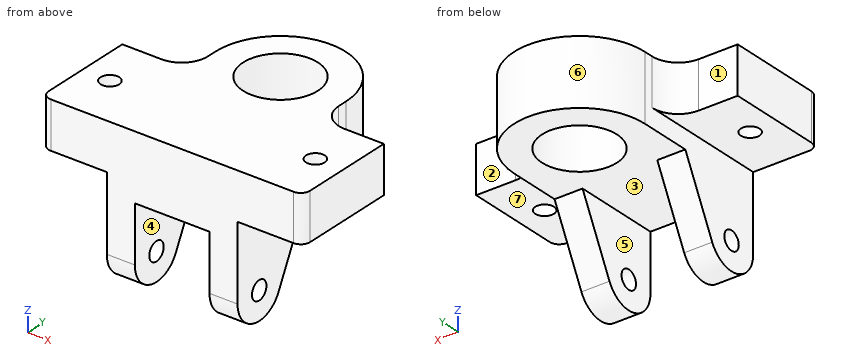
from build123d import *

# Parameters (mm, degrees)
SKETCH1_R           = 5
SKETCH1_R_2         = 20
BOSS_EXTRUDE1_DEPTH = 25
FILLET1_R           = 14
FILLET2_R           = 5
BOSS_EXTRUDE2_START = -10
SKETCH1_3_R         = 20
BOSS_EXTRUDE2_DEPTH = 10
SKETCH3_R           = 5
BOSS_EXTRUDE3_DEPTH = 15


with BuildPart() as part:
    # Sketch1 → Boss-Extrude1 (new body)
    with BuildSketch(Plane.XY):
        with BuildLine():
            Line((-70, 56), (-70, 0))
            Line((-70, 0), (70, 0))
            Line((70, 0), (70, 56))
            Line((70, 56), (35, 56))
            Line((35, 56), (35, 75))
            ThreePointArc((35, 75), (0, 110), (-35, 75))
            Line((-35, 75), (-35, 56))
            Line((-35, 56), (-70, 56))
        make_face()
        with Locations((-55, 28)):
            Circle(SKETCH1_R, mode=Mode.SUBTRACT)
        with Locations((0, 75)):
            Circle(SKETCH1_R_2, mode=Mode.SUBTRACT)
        with Locations((55, 28)):
            Circle(SKETCH1_R, mode=Mode.SUBTRACT)
    extrude(amount=BOSS_EXTRUDE1_DEPTH)

    # Fillet1
    fillet1_edges = [part.edges().sort_by_distance(p)[0] for p in [
        (-35, 56, 12.5),
        (35, 56, 12.5),
    ]]
    fillet(fillet1_edges, radius=FILLET1_R)

    # Fillet2
    fillet2_edges = [part.edges().sort_by_distance(p)[0] for p in [
        (-70, 0, 12.5),
        (70, 0, 12.5),
    ]]
    fillet(fillet2_edges, radius=FILLET2_R)

    # Sketch1_3 → Boss-Extrude2 (add)
    with BuildSketch(Plane.XY.offset(BOSS_EXTRUDE2_START)):
        with BuildLine():
            Line((-35, 56), (-35, 0))
            Line((-35, 0), (35, 0))
            Line((35, 0), (35, 56))
            Line((35, 56), (35, 75))
            ThreePointArc((35, 75), (0, 110), (-35, 75))
            Line((-35, 75), (-35, 56))
        make_face()
        with Locations((0, 75)):
            Circle(SKETCH1_3_R, mode=Mode.SUBTRACT)
    extrude(amount=BOSS_EXTRUDE2_DEPTH)

    # Sketch3 → Boss-Extrude3 (add)
    with BuildSketch(Plane(origin=(35, 0, 0), x_dir=(0, 0, -1), z_dir=(1, 0, 0))):
        with BuildLine():
            Line((10, 47), (10, 0))
            Line((10, 0), (40, 0))
            ThreePointArc((40, 0), (54.590100754, 11.517334354), (46.774992355, 28.382805333))
            Line((46.774992355, 28.382805333), (10, 47))
        make_face()
        with Locations((40, 15)):
            Circle(SKETCH3_R, mode=Mode.SUBTRACT)
    extrude(amount=-BOSS_EXTRUDE3_DEPTH)

    # Mirror1: part across plane


with BuildPart() as part_1:
    add(part.part)
    add(part.part.mirror(Plane(origin=(0, 0, 0), x_dir=(0, 0, 1), z_dir=(1, 0, 0))))


solid = part_1.part
Part model, mm, in its own coordinate system. Face numbers are marked on the shaded views. A direction names the side the tool comes from. Coordinates: 2 decimals unless noted, no trailing zeros. Order: outer loops, then holes, each group sorted by start corner. A loop starts at its lowest first (then second) coordinate and runs counter-clockwise, first axis right, second up.
(1) Tool access for the marked faces 1, 2, 3 and 4: list every direction of +Z, -Z, +X, -X, +Y, -Y with a clear straight run to the whole face (end or side of a thin tool).
Check sheet entries:
face 1: +Z, -Z, -X, +Y
face 2: +Z, -Z, +X, +Y
face 3: -Z, +Y
face 4: -Z, +Y, -Y
(2) Pull direction X, two halves, no side cores. Call the marked faces 5, 6 and 7: pulls with the +X half, pulls with the -X half, needs draft (parallel to the pull), parting line crosses it, or undercut.
Check sheet entries:
face 5: undercut
face 6: parting line crosses it
face 7: needs draft
(3) Slice it at D-D, the plane z = -3. Write the cut outline in (x, y), and give its area (3 significant figures).
Check sheet entries:
outline: (-35, 0) - (35, 0) - (35, 75) arc R35 ccw to (-35, 75) - close; hole circle Ø40 at (0, 75)
area: 5,920 mm2
(4) Slice it at B-B, the plane y = 15. Write the cut outline in (x, z).
Check sheet entries:
outline: (-70, 0) - (-35, 0) - (-35, -35) - (-20, -35) - (-20, -10) - (20, -10) - (20, -35) - (35, -35) - (35, 0) - (70, 0) - (70, 25) - (-70, 25) - close; (-35, -55) - (-20, -55) - (-20, -45) - (-35, -45) - close; (20, -55) - (35, -55) - (35, -45) - (20, -45) - close
(5) Pin check, flat tips, straight feed: pin 1 Ø10.5 at (x, z) = (64, 18.5) entering from +Y; pin 2 Ø10.5 at (x, y) = (58, 21) entering from -Z; pin 3 Ø13 at (y, z) = (15, -40) entering from +X. Stop position of each tip, or through.
Check sheet entries:
pin 1: stops at y = 56
pin 2: stops at z = 0
pin 3: stops at x = 35
(6) Slice it at A-A, the plane x = 55. Write the cut outline in (y, z).
Check sheet entries:
outline: (0, 0) - (23, 0) - (23, 25) - (0, 25) - close; (33, 0) - (56, 0) - (56, 25) - (33, 25) - close
(7) Slice it at C-C, the plane z = -13. Write the cut outline in (x, y).
Check sheet entries:
outline: (-35, 0) - (-20, 0) - (-20, 45.48) - (-35, 45.48) - close; (20, 0) - (35, 0) - (35, 45.48) - (20, 45.48) - close
(8) Probe L1, parallel to X at y = 28, z = 14.5; L2, parallel to Y at x = -55, z = 10.75; L3, parallel to Y at x = 0, z = 4. List the from-to ranges inside material, lowest first.
Check sheet entries:
L1: x = -70 to -60, -50 to 50, 60 to 70
L2: y = 0 to 23, 33 to 56
L3: y = 0 to 55, 95 to 110
